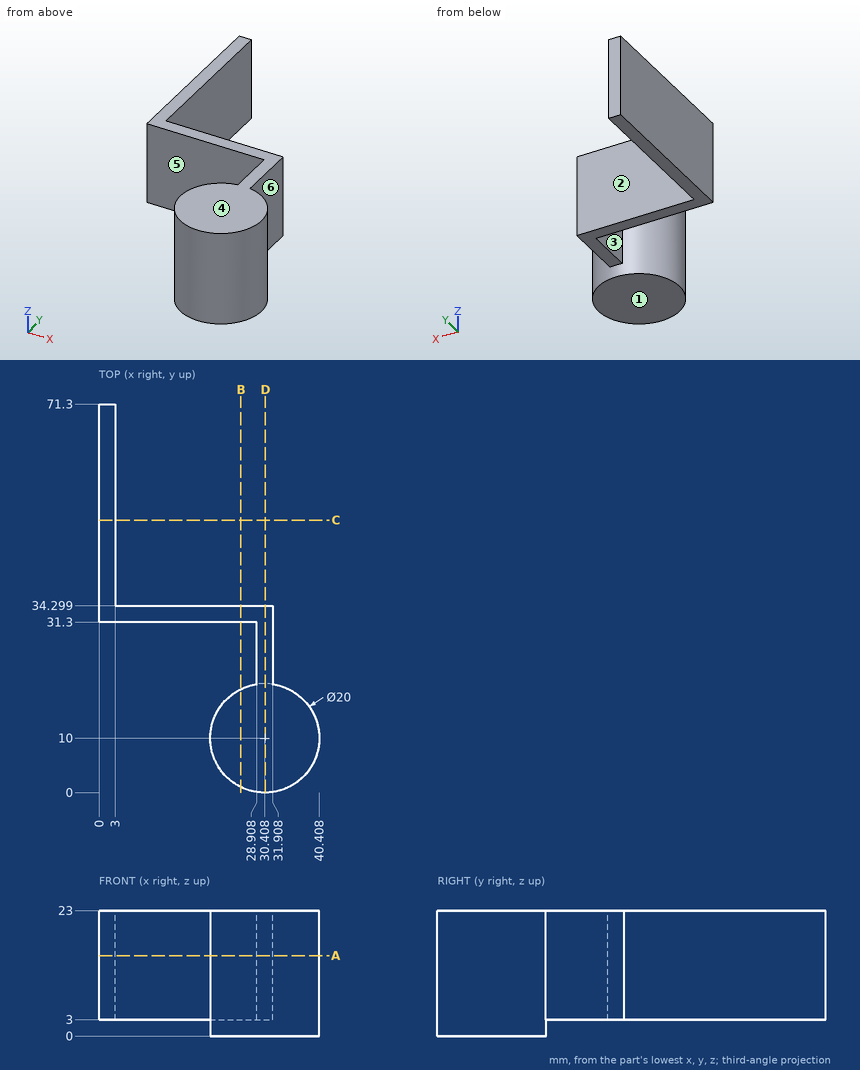
Here's the drawing with two shaded views (mm, measured from the low corner). I have some questions. A direction names the side the tool comes from. Round coordinates to 2 decimals unless told otherwise and drop trailing zeros. Write each loop counter-clockwise with the first axis right and the second up, starting at its lowest first coordinate (ties: lowest second). Pieces come first, ordered by that corner, then holes.
(1) Suppose I cut it at B-B on x = 26. Write out the boundary of the cut face in (y, z), and give its area (3 significant figures).
Findings below:
outline: (1.02, 0) - (18.98, 0) - (18.98, 23) - (1.02, 23) - close; (31.3, 3) - (34.3, 3) - (34.3, 23) - (31.3, 23) - close
area: 473 mm2
(2) For pin 1 (5 mm diameter, centred on x = 25, z = 8.5, fed in from -Y); pin 2 (6 mm diameter, centred on x = 33.5, z = 14, fed in from +Y); pin 3 (4 mm diameter, centred on y = 37.5, z = 13.5, fed in from -X); pin 4 (3 mm diameter, centred on x = 27, z = 6, fed in from -Y), each with a flat end and sliding along its axis, tell me the tip position at first contact or that it passes through.
Findings below:
pin 1: stops at y = 0.43
pin 2: stops at y = 34.3
pin 3: stops at x = 0
pin 4: stops at y = 0.18
(3) Suppose I cut it at C-C on y = 50. Write out the boundary of the cut face in (x, z).
Findings below:
outline: (0, 3) - (3, 3) - (3, 23) - (0, 23) - close
(4) Which directions (+Z, -Z, +X, -X, +Y, -Y) give clear straight access to the entire face, cutting with the end or side of a thin tool? Please do the marked faces 4, 5 and 6.
Findings below:
face 4: +Z, +X, -X, +Y, -Y
face 5: +Z, -Z, -X
face 6: +Z, -Z, +X, +Y
(5) If I drill on probe 1 along Y at (x, z) = (14, 16); probe 2 along X at (y, z) = (61.5, 11); probe 3 along Y at (x, z) = (22, 8.25) (1 decimal), over which ranges is the centre line in solid material (lowest first)?
Findings below:
probe 1: y = 31.3 to 34.3
probe 2: x = 0 to 3
probe 3: y = 4.6 to 15.4, 31.3 to 34.3
(6) Suppose I cut it at A-A on z = 14.75. Write out the boundary of the cut face in (x, y).
Findings below:
outline: (0, 31.3) - (28.91, 31.3) - (28.91, 19.89) arc R10 ccw (long way) to (31.91, 19.89) - (31.91, 34.3) - (3, 34.3) - (3, 71.3) - (0, 71.3) - close
(7) Thinking about a two-plate mould opening in Y: for the marked faces 1, 2 and 3, which applies, +Y half, -Y half, draft (parallel to the pull), parting line (faces both ways), or undercut?
Findings below:
face 1: draft
face 2: +Y half
face 3: undercut
(8) Suppose I cut it at D-D on x = 30.5. Write out the boundary of the cut face in (y, z), and give its area (3 significant figures).
Findings below:
outline: (0, 0) - (20, 0) - (20, 3) - (34.3, 3) - (34.3, 23) - (0, 23) - close
area: 746 mm2
